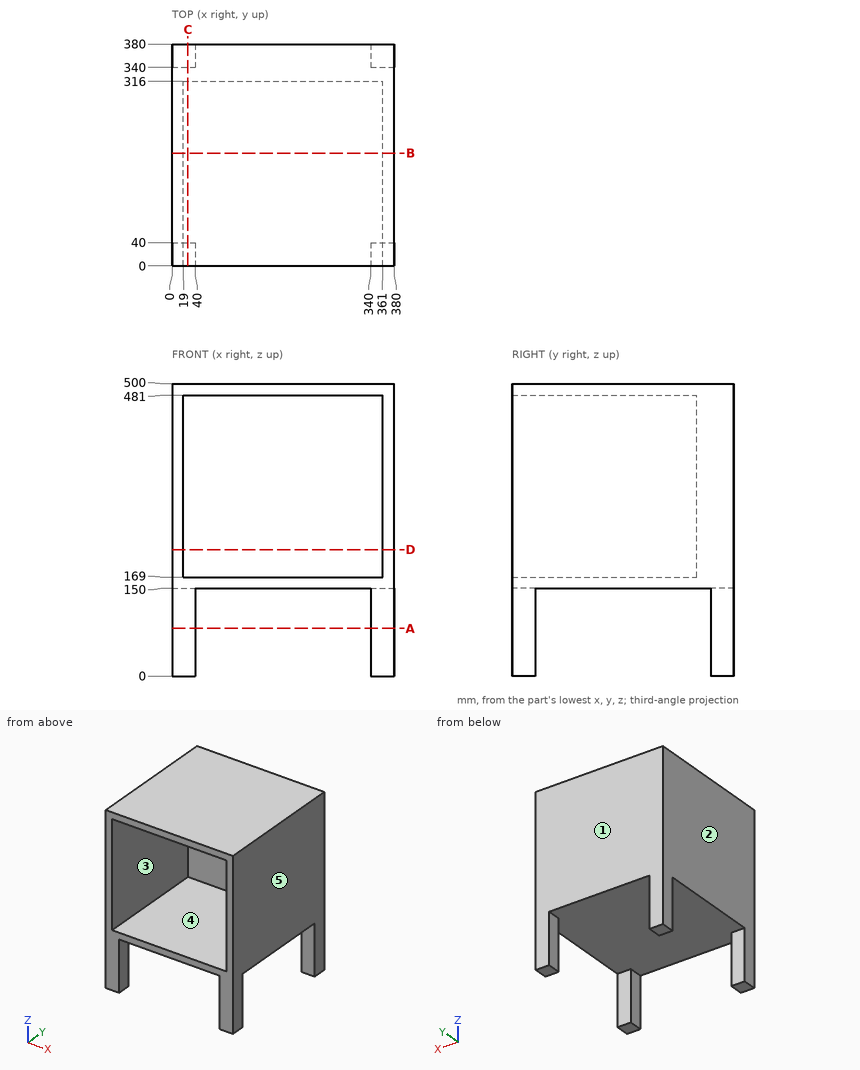
The figure shows three views and two pictorial views of one solid part (mm, origin at its lowest corner). Answer the questions. A direction names the side the tool comes from. Give positions to 0.01 mm unless a question says otherwise; leave off trailing zeros. Order: outer loops, then holes, each group sorted by start corner. A loop starts at its lowest first (then second) coordinate and runs counter-clockwise, first axis right, second up. Notation, with made-up numbers: (51.25, 65) -> (69.25, 65) arc R14 ccw to (69.25, 79) -> close; hole circle Ø11 at (34.5, 22). An arc over 180 degrees is marked (long way). Answer as CSV lines item,"result". Start each with the question number.
Q1. Given pin 1 (4 mm diameter, centred on x = 173, y = 99.5, fed in from -Z), flat-ended and moving along its own axis, determine where the tip first touches the part or whether it passes through.
Q2. Determine the mould class of the marked faces 1, 2 and 3 for opening direction X: pulls with the +X half, pulls with the -X half, needs draft (parallel to the pull), parting line crosses it, or undercut.
Q3. A cutting plane is placed at D-D (z = 216.5). Determine the outline of the cut face in (x, y).
Q4. Which of the six approach directions +Z, -Z, +X, -X, +Y, -Y give full straight-line access (tool end or side, diameter ignored) to the marked faces 4 and 5?
Q5. Find the intervals of material crossed by L1, parallel to Z at x = 104, y = 290; L2, parallel to Z at x = 352, y = 38; L3, parallel to Y at x = 77, z = 355, in increasing order.
Q6. A cutting plane is placed at B-B (y = 193). Determine the outline of the cut face in (x, z), then the cut area to 3 significant figures.
Q7. A cutting plane is placed at C-C (x = 27). Determine the outline of the cut face in (y, z), then the cut area to 3 significant figures.
Q8. A cutting plane is placed at A-A (z = 81.5). Determine the outline of the cut face in (x, y).
Results found:
1,pin 1,"z = 150"
2,face 1,"needs draft"
2,face 2,"pulls with the -X half"
2,face 3,"undercut"
3,outline,"(0, 0) -> (19, 0) -> (19, 316) -> (361, 316) -> (361, 0) -> (380, 0) -> (380, 380) -> (0, 380) -> close"
4,face 4,"-Y"
4,face 5,"+Z, -Z, +X, +Y, -Y"
5,L1,"150 to 169, 481 to 500"
5,L2,"0 to 169, 481 to 500"
5,L3,"316 to 380"
6,outline,"(0, 150) -> (380, 150) -> (380, 500) -> (0, 500) -> close; hole (19, 169) -> (361, 169) -> (361, 481) -> (19, 481) -> close"
6,area,"26,300 mm2"
7,outline,"(0, 0) -> (40, 0) -> (40, 150) -> (340, 150) -> (340, 0) -> (380, 0) -> (380, 500) -> (0, 500) -> (0, 481) -> (316, 481) -> (316, 169) -> (0, 169) -> close"
7,area,"46,400 mm2"
8,outline,"(0, 0) -> (40, 0) -> (40, 40) -> (0, 40) -> close; (0, 340) -> (40, 340) -> (40, 380) -> (0, 380) -> close; (340, 0) -> (380, 0) -> (380, 40) -> (340, 40) -> close; (340, 340) -> (380, 340) -> (380, 380) -> (340, 380) -> close"
